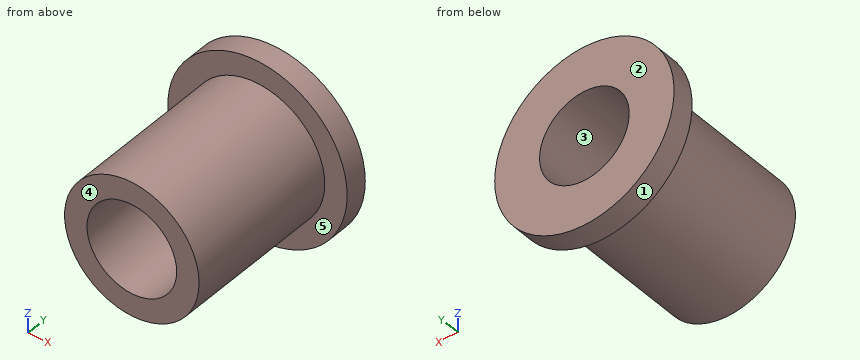
from build123d import *

# Parameters (mm, degrees)
F0_R     = 6.35
F1_DEPTH = 1.6002
F2_R     = 4.7625
F3_DEPTH = 11.0998
F4_R     = 3.175
F5_DEPTH = 19.05


with BuildPart() as f1:
    # F0 (on Front) → F1 (new body)
    with BuildSketch(Plane.XZ):
        Circle(F0_R)
    extrude(amount=-F1_DEPTH)

    # F2 (on face) → F3 (join)
    with BuildSketch(Plane.XZ):
        Circle(F2_R)
    extrude(amount=F3_DEPTH)

    # F4 (on face) → F5 (cut, symmetric)
    with BuildSketch(Plane.XZ):
        Circle(F4_R)
    extrude(amount=F5_DEPTH, both=True, mode=Mode.SUBTRACT)


solid = f1.part
Can you work these out from the model? Positions are in its coordinate system, mm. Face numbers are marked on the shaded views. A direction names the side the tool comes from. Give positions to 0.01 mm unless a question says otherwise; leave off trailing zeros. Order: outer loops, then holes, each group sorted by start corner. A loop starts at its lowest first (then second) coordinate and runs counter-clockwise, first axis right, second up. Notation, with made-up numbers: M 70.25,81.5 L 88.25,81.5 A19 ccw 88.25,92.5 Z; hole C 43.5,-15 d5. An arc over 180 degrees is marked long. Use one line per item in the form item = value.
Item 1: For the marked faces 4 and 5, which set-ups out of +Z, -Z, +X, -X, +Y, -Y let a thin tool reach every point of the face, with its end or its side?
Values follow:
face_4 = +Z, -Z, +X, -X, -Y
face_5 = -Y
Item 2: If we section it at D-D, the plane z = 4.25: Write out the boundary of the cut face in (x, y).
Values follow:
outline = M -4.72,0 L -2.15,0 L -2.15,-11.1 L 2.15,-11.1 L 2.15,0 L 4.72,0 L 4.72,1.6 L -4.72,1.6 Z
Item 3: Will these pins go through, and if not, where does the flat tip stop? pin 1 Ø3 at (x, y) = (4, -3) entering from +Z; pin 2 Ø2 at (y, z) = (-7.5, 2) entering from +X; pin 3 Ø5 at (x, y) = (3, -8.5) entering from -Z.
Values follow:
pin_1 = 4.05
pin_2 = 4.66
pin_3 = -4.74
Item 4: If I drill on line 1 along Z through (x, y) = (0, -2.25) (1 decimal); line 2 along Z through (x, y) = (1.75, -6.5); line 3 along Y through (x, z) = (-5.25, -2.5), over which ranges is the centre line in solid material (lowest first)? Write a range as [from, to].
Values follow:
line_1 = [-4.8, -3.2], [3.2, 4.8]
line_2 = [-4.43, -2.65], [2.65, 4.43]
line_3 = [0, 1.6]
Item 5: Thinking about a two-plate mould opening in Z: for the marked faces 1, 2 and 3, which applies, pulls with the +Z half, pulls with the -Z half, needs draft (parallel to the pull), parting line crosses it, or undercut?
Values follow:
face_1 = parting line crosses it
face_2 = needs draft
face_3 = undercut
